Check sheet for the modelled part. Datum: model origin and axes. Units: mm. Coordinates: 2 decimals unless noted, no trailing zeros. Loops run counter-clockwise (first coordinate to the right, second up) from the corner with the lowest first, then second, coordinate; pieces in that order, holes last. Notation, with made-up numbers: (7, 11.5) - (63, 11.5) arc R21 cw to (63, 31.5) - close; hole circle Ø10 at (0.25, 71.25). An arc over 180 degrees is marked (long way). Use a Markdown table: item, result. Add a question column.
1) Thickness scan on line 1 (Y direction, x = -105.5, z = 1.5); line 2 (Y direction, x = -117.5, z = 2); line 3 (Y direction, x = -63.5, z = 7.5) (3 decimals). Record the ranges inside material, lowest first.
2) Go/stop test with flat-tipped pins: P1, Ø7.5, axis at x = -116.74, y = 11.85, coming from the -Z side (3 decimals); P2, Ø1, axis at y = 104, z = 3, coming from the -X side; P3, Ø1, axis at x = -33, z = 8, coming from the +Y side. Record where each tip stops, or that it passes through.
3) Sectioned sample at B-B, the plane x = -32.5. Enter the section's corners in (y, z) (3 decimals), then the cut area to 3 significant figures.
4) Sectioned sample at A-A, the plane x = -63.5. State how many separate pieces and enclosed holes the cut face has, then the cut area to 3 significant figures.
5) Sectioned sample at C-C, the plane y = 37. Enter the section's corners in (x, z) (3 decimals).
from build123d import *

# Parameters (mm, degrees)
F0_R     = 3.175
F1_DEPTH = 9.525
F2_R     = 5.08
F3_SIZE  = 2.54
F5_DEPTH = 3.175
F6_R     = 7.4295
F7_DEPTH = 3.175


with BuildPart() as f1:
    # F0 (on Top) → F1 (new body)
    with BuildSketch(Plane.XY):
        Polygon((25.4, 175.976362), (-152.4, 175.976362), (-139.7, 87.988181), (-127, 0), (0, 0), align=None)
        with Locations((-116.737792, 11.849777)):
            Circle(F0_R, mode=Mode.SUBTRACT)
        with BuildLine():
            ThreePointArc((-126.901293, 87.988181), (-130.076293, 84.813181), (-133.251293, 87.988181))
            ThreePointArc((-133.251293, 87.988181), (-130.076293, 91.163181), (-126.901293, 87.988181))
        make_face(mode=Mode.SUBTRACT)
        with Locations((-63.5, 9.525)):
            Circle(F0_R, mode=Mode.SUBTRACT)
        with Locations((-10.262208, 11.849777)):
            Circle(F0_R, mode=Mode.SUBTRACT)
        with Locations((3.076293, 87.988181)):
            Circle(F0_R, mode=Mode.SUBTRACT)
        with Locations((-137.603178, 163.161938)):
            Circle(F0_R, mode=Mode.SUBTRACT)
        Polygon((-110.502216, 19.05), (-120.452585, 87.988181), (-130.402955, 156.926362), (3.402955, 156.926362), (-16.497784, 19.05), align=None, mode=Mode.SUBTRACT)
        with Locations((-63.5, 166.451362)):
            Circle(F0_R, mode=Mode.SUBTRACT)
        with Locations((10.603178, 163.161938)):
            Circle(F0_R, mode=Mode.SUBTRACT)
    extrude(amount=F1_DEPTH)

    # F2
    f2_edges = [f1.edges().sort_by_distance(p)[0] for p in [
        (-152.4, 175.976362, 4.7625),
        (-130.402955, 156.926362, 4.7625),
        (25.4, 175.976362, 4.7625),
        (3.402955, 156.926362, 4.7625),
        (-127, 0, 4.7625),
        (0, 0, 4.7625),
        (-16.497784, 19.05, 4.7625),
        (-110.502216, 19.05, 4.7625),
    ]]
    fillet(f2_edges, radius=F2_R)

    # F3
    f3_edges = [f1.edges().sort_by_distance(p)[0] for p in [
        (-63.5, 0, 9.525),
    ]]
    chamfer(f3_edges, length=F3_SIZE)

    # F4 (on face) → F5 (cut)
    with BuildSketch(Plane(origin=(0, 0, 0), x_dir=(1, 0, 0), z_dir=(0, 0, -1))):
        with BuildLine():
            ThreePointArc((-3.299557, -21.59), (-9.257451, -10.689583), (-20.897193, -6.35))
            Line((-20.897193, -6.35), (-106.102807, -6.35))
            ThreePointArc((-106.102807, -6.35), (-117.742549, -10.689583), (-123.700443, -21.59))
            Line((-123.700443, -21.59), (-142.134712, -149.306362))
            ThreePointArc((-142.134712, -149.306362), (-137.977493, -163.486104), (-124.537076, -169.626362))
            Line((-124.537076, -169.626362), (-2.462924, -169.626362))
            ThreePointArc((-2.462924, -169.626362), (10.977493, -163.486104), (15.134712, -149.306362))
            Line((15.134712, -149.306362), (-3.299557, -21.59))
        make_face()
    extrude(amount=-F5_DEPTH, mode=Mode.SUBTRACT)

    # F6 (on face) → F7 (cut, through all)
    with BuildSketch(Plane(origin=(0, 0, 0), x_dir=(1, 0, 0), z_dir=(0, 0, -1))):
        with Locations((-116.737792, -11.849777)):
            Circle(F6_R)
        with Locations((-63.5, -9.525)):
            Circle(F6_R)
        with Locations((-10.262208, -11.849777)):
            Circle(F6_R)
        with Locations((3.076293, -87.988181)):
            Circle(F6_R)
        with Locations((-63.5, -166.451362)):
            Circle(F6_R)
        with Locations((-137.603178, -163.161938)):
            Circle(F6_R)
        with Locations((10.603178, -163.161938)):
            Circle(F6_R)
        with Locations((-130.076293, -87.988181)):
            Circle(F6_R)
    extrude(amount=-F7_DEPTH, mode=Mode.SUBTRACT)


solid = f1.part
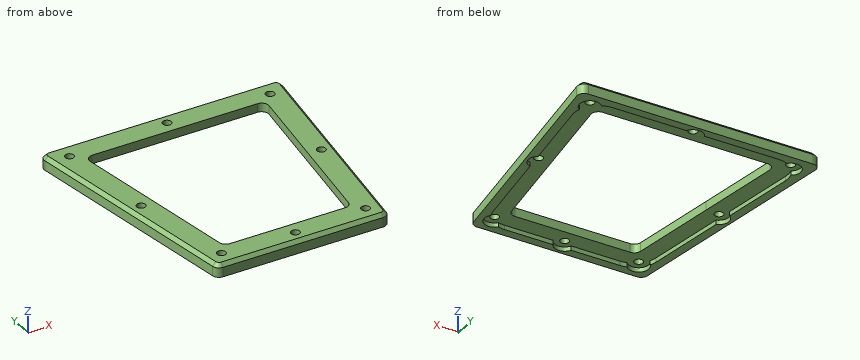
Solved:
| question | item | result |
|---|---|---|
| 1 | line 1 | y = 0 to 6.35, 169.63 to 175.98 |
| 1 | line 2 | y = 0 to 4.46, 169.63 to 175.98 |
| 1 | line 3 | y = 0.515 to 6.35, 12.7 to 19.05, 156.926 to 163.276, 169.626 to 175.461 |
| 2 | P1 | stops at z = 3.175 |
| 2 | P2 | stops at x = -142.08 |
| 2 | P3 | stops at y = 175.46 |
| 3 | outline | (0, 0) - (6.35, 0) - (6.35, 3.175) - (19.05, 3.175) - (19.05, 9.525) - (2.54, 9.525) - (0, 6.985) - close; (156.926, 3.175) - (169.626, 3.175) - (169.626, 0) - (175.976, 0) - (175.976, 6.985) - (173.436, 9.525) - (156.926, 9.525) - close |
| 3 | area | 276 mm2 |
| 4 | separate pieces | 4 |
| 4 | enclosed holes | 0 |
| 4 | area | 168 mm2 |
| 5 | outline | (-132.34, 0) - (-125.925, 0) - (-125.925, 3.175) - (-113.093, 3.175) - (-113.093, 9.525) - (-129.774, 9.525) - (-132.34, 6.985) - close; (-13.907, 3.175) - (-1.075, 3.175) - (-1.075, 0) - (5.34, 0) - (5.34, 6.985) - (2.774, 9.525) - (-13.907, 9.525) - close |
